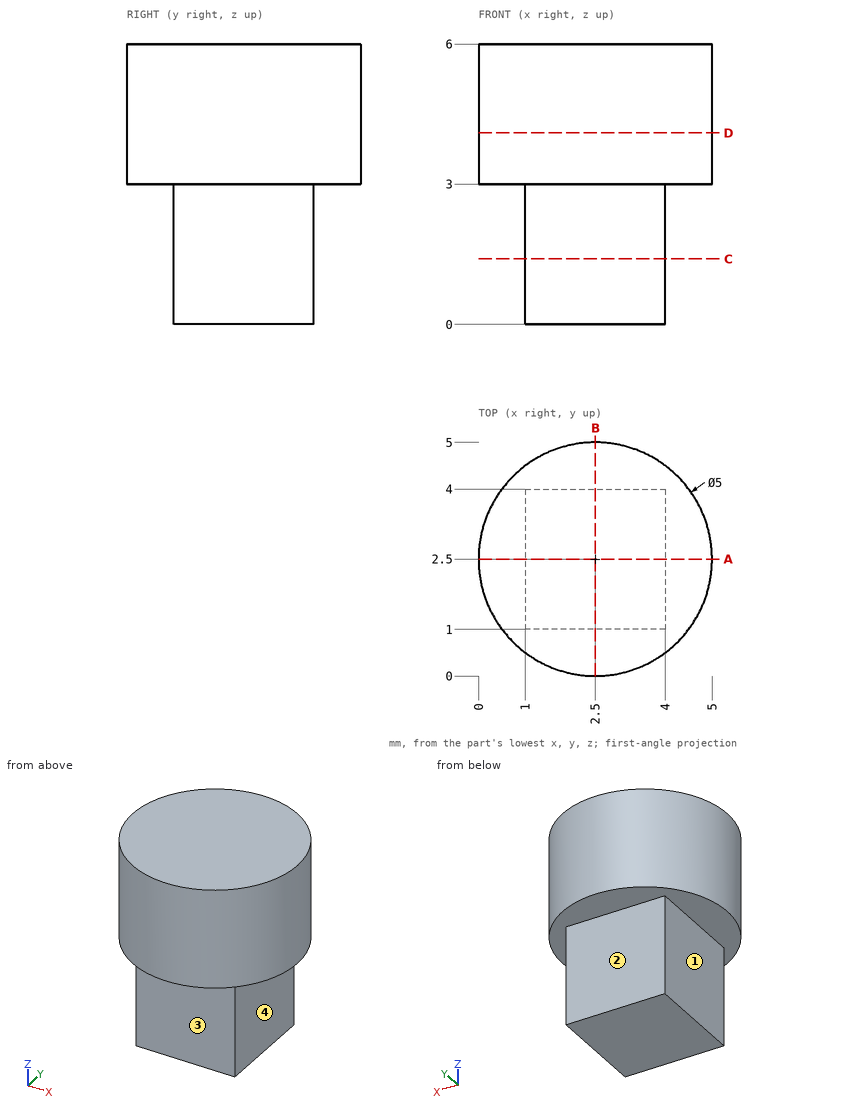
The drawing under review shows one solid part. Ordinate dimensions are in mm from its lowest x, y, z. A direction names the side the tool comes from. Give positions to 0.01 mm unless a question says otherwise; leave off trailing zeros. Loops run counter-clockwise (first coordinate to the right, second up) from the corner with the lowest first, then second, coordinate; pieces in that order, holes last. Notation, with made-up numbers: M 63,36 L 98,36 A10 cw 98,41 Z; hole C -39,-23.5 d10. An arc over 180 degrees is marked long. One line per question, with ' | ' between items. Start each with the question number.
1. Add section C-C (z = 1.4). Write out the cut boundary in (x, y), plus the area to 3 significant figures.
2. Insertion check: P1, Ø1.5, axis at y = 3, z = 1, coming from the -X side; P2, Ø1.5, axis at x = 2.5, z = 1, coming from the -Y side; P3, Ø1.5, axis at x = 2, z = 1, coming from the +Y side. Each pin has a flat end and moves straight along its axis. Give the tip position at first contact, or say it passes through.
3. Add section A-A (y = 2.5). Write out the cut boundary in (x, z), plus the area to 3 significant figures.
4. For the marked faces 1, 2, 3 and 4, list the 3-axis set-ups (+Z, -Z, +X, -X, +Y, -Y) from which the entire face can be reached by the end or side of a thin tool; tool diameter is ignored.
5. Add section D-D (z = 4.1). Write out the cut boundary in (x, y), plus the area to 3 significant figures.
6. To check wall thickness, follow L1, parallel to Z at x = 1.45, y = 4.5; L2, parallel to Y at x = 3.3, z = 0.4. State the ranges of each line that lie inside material, in increasing order.
Worked out:
1) outline: M 1,1 L 4,1 L 4,4 L 1,4 Z | area: 9.00 mm²
2) P1: stops at x = 1 | P2: stops at y = 1 | P3: stops at y = 4
3) outline: M 0,3 L 1,3 L 1,0 L 4,0 L 4,3 L 5,3 L 5,6 L 0,6 Z | area: 24.0 mm²
4) face 1: -Z, -X, +Y, -Y | face 2: -Z, +X, -X, +Y | face 3: -Z, +X, -X, -Y | face 4: -Z, +X, +Y, -Y
5) outline: C 2.5,2.5 d5 | area: 19.6 mm²
6) L1: z = 3 to 6 | L2: y = 1 to 4
